```python
from build123d import *

# Parameters (mm, degrees)
EXTRUDE_1_DEPTH     = 4
SWEEP_4_OUTLINE_R   = 0.25
SWEEP_4_ANGLE       = 90
SWEEP_START         = -0.5
SWEEP_4_2_OUTLINE_R = 0.25
SWEEP_4_2_DEPTH     = 1.5000001
SWEEP_START_2       = -7.0000001
SWEEP_4_3_OUTLINE_R = 0.25
SWEEP_4_3_DEPTH     = 2.0000001
SWEEP_4_4_OUTLINE_R = 0.25
SWEEP_4_4_DEPTH     = 1.5000001
SWEEP_4_5_OUTLINE_R = 0.25
SWEEP_4_5_DEPTH     = 2.0000001
FILLET_1_R          = 0.5
FILLET_2_R          = 0.5


with BuildPart() as part:
    # Sketch 1 → Extrude 1 (new body)
    with BuildSketch(Plane(origin=(0, 0, 0), x_dir=(1, 0, 0), z_dir=(0, 1, 0))):
        with BuildLine():
            Line((-5, 3.85), (5, 3.85))
            ThreePointArc((5, 3.85), (5.707106781, 3.557106781), (6, 2.85))
            Line((6, 2.85), (6, -2.85))
            ThreePointArc((6, -2.85), (5.707106781, -3.557106781), (5, -3.85))
            Line((5, -3.85), (-5, -3.85))
            ThreePointArc((-5, -3.85), (-5.707106781, -3.557106781), (-6, -2.85))
            Line((-6, -2.85), (-6, 2.85))
            ThreePointArc((-6, 2.85), (-5.707106781, 3.557106781), (-5, 3.85))
        make_face()
    extrude(amount=EXTRUDE_1_DEPTH)



with BuildPart() as body_2:
    # Sweep 4: read off the stored shape, not the designer's step
    # Sweep 4 outline → Sweep 4 (revolve)
    with BuildSketch(Plane(origin=(-7, 1, 0), x_dir=(0, 1, 0), z_dir=(1, 0, 0))):
        with Locations((1, -2.5)):
            Circle(SWEEP_4_OUTLINE_R)
        with Locations((1, 2.5)):
            Circle(SWEEP_4_OUTLINE_R)
    revolve(axis=Axis((-7, 1, 0), (0, 0, 1)), revolution_arc=SWEEP_4_ANGLE)

    # Sweep 4 2 outline → Sweep 4 2 (add)
    with BuildSketch(Plane(origin=(0, 0, 0), x_dir=(1, 0, 0), z_dir=(0, 1, 0)).offset(SWEEP_START)):
        with Locations((-8, 2.5)):
            Circle(SWEEP_4_2_OUTLINE_R)
    extrude(amount=SWEEP_4_2_DEPTH)


with BuildPart() as part_1:
    add(part.part)

    add(body_2.part)  # Sweep 4 3 merges body 2
    # Sweep 4 3 outline → Sweep 4 3 (add)
    with BuildSketch(Plane.YZ.offset(SWEEP_START_2)):
        with Locations((2, -2.5)):
            Circle(SWEEP_4_3_OUTLINE_R)
    extrude(amount=SWEEP_4_3_DEPTH)

    # Sweep 4 4 outline → Sweep 4 4 (add)
    with BuildSketch(Plane(origin=(0, 0, 0), x_dir=(1, 0, 0), z_dir=(0, 1, 0)).offset(SWEEP_START)):
        with Locations((-8, -2.5)):
            Circle(SWEEP_4_4_OUTLINE_R)
    extrude(amount=SWEEP_4_4_DEPTH)

    # Sweep 4 5 outline → Sweep 4 5 (add)
    with BuildSketch(Plane.YZ.offset(SWEEP_START_2)):
        with Locations((2, 2.5)):
            Circle(SWEEP_4_5_OUTLINE_R)
    extrude(amount=SWEEP_4_5_DEPTH)

    # Fillet 1
    fillet_1_edges = [part_1.edges().sort_by_distance(p)[0] for p in [
        (-5.707106781, 4, 3.557106781),
        (0, 4, 3.85),
        (5.707106781, 4, 3.557106781),
        (6, 4, 0),
        (5.707106781, 4, -3.557106781),
        (0, 4, -3.85),
        (-5.707106781, 4, -3.557106781),
        (-6, 4, 0),
    ]]
    fillet(fillet_1_edges, radius=FILLET_1_R)

    # Fillet 2
    fillet_2_edges = [part_1.edges().sort_by_distance(p)[0] for p in [
        (0, 0, 3.85),
        (-5.707106781, 0, 3.557106781),
        (-6, 0, 0),
        (-5.707106781, 0, -3.557106781),
        (0, 0, -3.85),
        (5.707106781, 0, -3.557106781),
        (6, 0, 0),
        (5.707106781, 0, 3.557106781),
    ]]
    fillet(fillet_2_edges, radius=FILLET_2_R)


solid = part_1.part
```
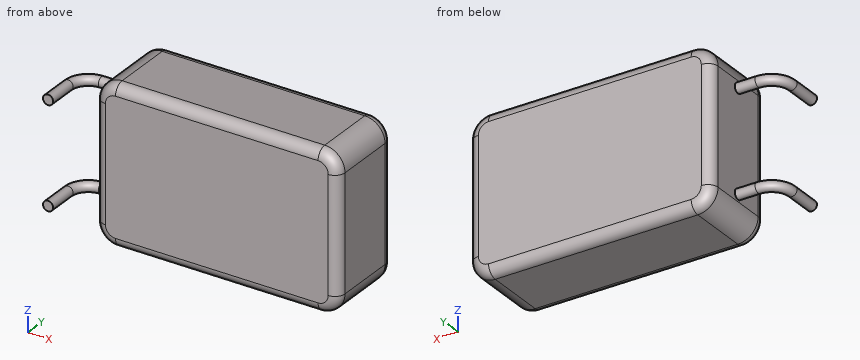
Here's how the part is built. I have some questions about the finished solid (model axes, mm). Give positions to 0.01 mm unless a question says otherwise; leave off trailing zeros. Order: outer loops, then holes, each group sorted by start corner. A loop starts at its lowest first (then second) coordinate and runs counter-clockwise, first axis right, second up. Notation, with made-up numbers: M 25,-4.5 L 69,-4.5 A25 cw 69,29.5 Z; hole C 65.25,4.25 d3. An arc over 180 degrees is marked long. Use a Markdown table: item, result. Add a question column.
1. Suppose I cut it at B-B (x = 1). List the corners of the cut face in (y, z) for me, and give its area (3 significant figures).
2. Suppose I cut it at C-C (z = 2.5). List the corners of the cut face in (x, y) for me.
3. Suppose I cut it at A-A (z = -2). List the corners of the cut face in (x, y) for me, and give its area (3 significant figures).
4. I need wall thicknesses on probe 1 along X at (y, z) = (1.15, -1.5); probe 2 along Y at (x, z) = (-3.25, -2.75); probe 3 along Z at (x, y) = (-3.75, 0.2). Which ranges of each line are inside material? Lowest first, please. Write a range as from..to.
5. Suppose I cut it at D-D (y = 1.2). Give the number of separate pieces and of enclosed holes in the cut face, and give its area (3 significant figures).
6. For pin 1 Ø2.5 at (y, z) = (2, -0.5) entering from -X, with a flat end and sliding along its axis, tell me the tip position at first contact or that it passes through.
Results list:
| question | item | result |
|---|---|---|
| 1 | outline | M 0,-3.35 A0.5 ccw 0.5,-3.85 L 3.5,-3.85 A0.5 ccw 4,-3.35 L 4,3.35 A0.5 ccw 3.5,3.85 L 0.5,3.85 A0.5 ccw 0,3.35 Z |
| 1 | area | 30.6 mm² |
| 2 | outline | M -8.25,-0.5 L -7.75,-0.5 L -7.75,1 A0.75 cw -7,1.75 L -6,1.75 L -6,0.5 A0.5 ccw -5.5,0 L 5.5,0 A0.5 ccw 6,0.5 L 6,3.5 A0.5 ccw 5.5,4 L -5.5,4 A0.5 ccw -6,3.5 L -6,2.25 L -7,2.25 A1.25 ccw -8.25,1 Z |
| 3 | outline | M -6,0.5 A0.5 ccw -5.5,0 L 5.5,0 A0.5 ccw 6,0.5 L 6,3.5 A0.5 ccw 5.5,4 L -5.5,4 A0.5 ccw -6,3.5 Z |
| 3 | area | 47.8 mm² |
| 4 | probe 1 | x = -6..6 |
| 4 | probe 2 | y = 0..4 |
| 4 | probe 3 | z = -3.75..3.75 |
| 5 | separate pieces | 3 |
| 5 | enclosed holes | 0 |
| 5 | area | 91.9 mm² |
| 6 | pin 1 | stops at x = -6 |
